from build123d import *

# Parameters (mm, degrees)
SKIZZE1_R                       = 40
AUFSATZ_LINEAR_AUSTRAGEN1_DEPTH = 50
SKIZZE2_R                       = 31.5
SKIZZE2_R_2                     = 15.75
SKIZZE2_R_3                     = 3
AUFSATZ_LINEAR_AUSTRAGEN2_DEPTH = 6.2
FASE1_SIZE                      = 1


with BuildPart() as part:
    # Skizze1 → Aufsatz-Linear austragen1 (new body)
    with BuildSketch(Plane.XY):
        Circle(SKIZZE1_R)
    extrude(amount=AUFSATZ_LINEAR_AUSTRAGEN1_DEPTH)

    # Skizze2 → Aufsatz-Linear austragen2 (add)
    with BuildSketch(Plane.XY.offset(50)):
        with Locations(Location((0, 0, 0), (0, 0, 180))):
            Circle(SKIZZE2_R)
        with Locations(Location((0, 0, 0), (0, 0, 180))):
            Circle(SKIZZE2_R_2, mode=Mode.SUBTRACT)
        with Locations(Location((0, 25, 0), (0, 0, 180))):
            Circle(SKIZZE2_R_3, mode=Mode.SUBTRACT)
        with Locations(Location((17.67766953, 17.67766953, 0), (0, 0, 180))):
            Circle(SKIZZE2_R_3, mode=Mode.SUBTRACT)
        with Locations(Location((17.67766953, -17.67766953, 0), (0, 0, 180))):
            Circle(SKIZZE2_R_3, mode=Mode.SUBTRACT)
        with Locations(Location((-17.67766953, -17.67766953, 0), (0, 0, 180))):
            Circle(SKIZZE2_R_3, mode=Mode.SUBTRACT)
        with Locations(Location((-17.67766953, 17.67766953, 0), (0, 0, 180))):
            Circle(SKIZZE2_R_3, mode=Mode.SUBTRACT)
    extrude(amount=AUFSATZ_LINEAR_AUSTRAGEN2_DEPTH)

    # Fase1
    fase1_edges = [part.edges().sort_by_distance(p)[0] for p in [
        (31.5, 0, 56.2),
        (15.75, 0, 56.2),
        (3, 25, 56.2),
        (20.67766953, 17.67766953, 56.2),
        (20.67766953, -17.67766953, 56.2),
        (-14.67766953, -17.67766953, 56.2),
        (-14.67766953, 17.67766953, 56.2),
        (-40, 0, 50),
    ]]
    chamfer(fase1_edges, length=FASE1_SIZE)


solid = part.part
Check sheet for the modelled part. Datum: model origin and axes. Units: mm. A direction names the side the tool comes from. Coordinates: 2 decimals unless noted, no trailing zeros. Loops run counter-clockwise (first coordinate to the right, second up) from the corner with the lowest first, then second, coordinate; pieces in that order, holes last. Notation, with made-up numbers: (32.25, 70) -> (41.25, 70) arc R27 ccw to (41.25, 97) -> close; hole circle Ø8 at (-13.75, 35.5). An arc over 180 degrees is marked (long way). Write item = value, one per line. Start each with the question number.
1. Material ranges on line 1 (Y direction, x = 0, z = 52.85); line 2 (Z direction, x = 15.5, y = -31); line 3 (X direction, y = 14, z = 44), recorded low to high.
2. Section check C-C on z = 35.5. Record the cut outline in (x, y), then the cut area to 3 significant figures.
3. Section check B-B on y = 0. Record the cut outline in (x, z), then the cut area to 3 significant figures.
4. Draft check along X on faces 1 (the cylindrical face through (-8.67, -39.05, 24.16)), 2 (the cylindrical face through (2.05, -15.616, 52.564)), 3 (the flat face through (3, 32, 50)). Enter one of: released by +X, released by -X, zero draft, split by the parting line, or undercut.
5. Section check A-A on x = 0. Record the cut outline in (y, z), then the cut area to 3 significant figures.
6. Tool access check on faces 4 (the cylindrical face through (-17, 20.6, 52.6)), 5 (the flat face through (-1, 1, 0)). Record the directions out of +Z, -Z, +X, -X, +Y, -Y that give a thin tool (end or side, any length) a straight path to the whole face; none if there is none.
7. Depth check by flat-ended pin: P1, Ø1.5, axis at y = -20, z = 20, coming from the -X side; P2, Ø5, axis at x = 16.5, y = -19, coming from the +Z side; P3, Ø1, axis at x = -12.5, z = 45.5, coming from the +Y side; P4, Ø5.5, axis at x = -17.68, y = -17.68, coming from the +Z side. Enter the tip coordinate at first touch or a pass-through.
Responses:
q1.line_1 = -31.5 to -15.75, 15.75 to 22, 28 to 31.5
q1.line_2 = 0 to 50
q1.line_3 = -37.47 to 37.47
q2.outline = circle Ø80 at (0, 0)
q2.area = 5,030 mm2
q3.outline = (-40, 0) -> (40, 0) -> (40, 49) -> (39, 50) -> (31.5, 50) -> (31.5, 55.2) -> (30.5, 56.2) -> (16.75, 56.2) -> (15.75, 55.2) -> (15.75, 50) -> (-15.75, 50) -> (-15.75, 55.2) -> (-16.75, 56.2) -> (-30.5, 56.2) -> (-31.5, 55.2) -> (-31.5, 50) -> (-39, 50) -> (-40, 49) -> close
q3.area = 4,190 mm2
q4.face_1 = split by the parting line
q4.face_2 = undercut
q4.face_3 = zero draft
q5.outline = (-40, 0) -> (40, 0) -> (40, 49) -> (39, 50) -> (31.5, 50) -> (31.5, 55.2) -> (30.5, 56.2) -> (29, 56.2) -> (28, 55.2) -> (28, 50) -> (22, 50) -> (22, 55.2) -> (21, 56.2) -> (16.75, 56.2) -> (15.75, 55.2) -> (15.75, 50) -> (-15.75, 50) -> (-15.75, 55.2) -> (-16.75, 56.2) -> (-30.5, 56.2) -> (-31.5, 55.2) -> (-31.5, 50) -> (-39, 50) -> (-40, 49) -> close
q5.area = 4,150 mm2
q6.face_4 = +Z
q6.face_5 = -Z, +X, -X, +Y, -Y
q7.P1 = -35.06
q7.P2 = 56.2
q7.P3 = 38.16
q7.P4 = 50
